Autodesk Inventor part; units mm, degrees
ref_plane "YZ Plane" through (0, 0, 0) normal (1, 0, 0) x (0, 1, 0)
ref_plane "XZ Plane" through (0, 0, 0) normal (0, 1, 0) x (-1, 0, 0)
ref_plane "XY Plane" through (0, 0, 0) normal (0, 0, 1) x (1, 0, 0)
sketch "Sketch1" plane through (0, 0, 0) normal (0, 0, 1) x (1, 0, 0)
  line L0 (0, 0) -> (22, 0)
  line L1 (22, 0) -> (22, 5)
  line L2 (22, 5) -> (0, 5)
  line L3 (0, 5) -> (0, 0)
  line L4 (22, 0) -> (13, 0)
  line L5 (13, 0) -> (13, 4)
  line L6 (13, 4) -> (22, 4)
  line L7 (22, 4) -> (22, 0)
  line L8 (13, 4) -> (13, 5)
  line L9 (22, 0) -> (0, 0)
  line L10 (0, 0) -> (0, 2.6)
  line L11 (0, 2.6) -> (22, 2.6)
  line L12 (22, 2.6) -> (22, 0)
  dimension "d0" = 22
  dimension "d1" = 5
  dimension "d2" = 9
  dimension "d3" = 4
  dimension "d4" = 2.6
revolve "Revolution1" add sketch "Sketch1" angle 360 about axis through (0, 0, 0) along (1, 0, 0) contours L3 L2 L8 L5 L11 | L5 L6 L1 L11
chamfer "Chamfer1" distance 1 angle 45 3 edges at (22, -2.6, 0) (0, -2.6, 0) (0, -5, 0)
properties part number "Vezetőhüvely"
Geometry check sheet. Reference: the model listing, model coordinates, mm. Give positions to 0.01 mm unless a question says otherwise; leave off trailing zeros. Order: outer loops, then holes, each group sorted by start corner. A loop starts at its lowest first (then second) coordinate and runs counter-clockwise, first axis right, second up. Notation, with made-up numbers: (63.5, -18.75) -> (81.5, -18.75) arc R20 cw to (81.5, 13.25) -> close; hole circle Ø5 at (56.25, 86). An arc over 180 degrees is marked (long way). Write each question's results on one line, items separated by ' | '. Start each with the question number.
(1) Scan lines: line 1 (Z direction, x = 6.75, y = 0); line 2 (Z direction, x = 13.5, y = 0); line 3 (Y direction, x = 10, z = 0.5). Record each from-to range of solid material in increasing order.
(2) Sectioned sample at D-D (x = 17.5). Enter the section's corners in (y, z).
(3) Sectioned sample at C-C (x = 4.25). Enter the section's corners in (y, z), plus the area to 3 significant figures.
(4) Sectioned sample at A-A (y = 0). Enter the section's corners in (x, z), plus the area to 3 significant figures.
(5) Mould release check, pull along Z, two halves, no side actions. Record for faces 1 (the face through (11.14, -0.338, 2.578)), 2 (the face through (6.92, -1.08, 4.88)): pulls with the +Z half, pulls with the -Z half, needs draft (parallel to the pull), parting line crosses it, or undercut.
(6) Gauge pin test, flat ends, axial feed: P1, Ø4, axis at x = 18, z = 1, coming from the -Y side; P2, Ø6, axis at x = 16.5, y = 2.5, coming from the +Z side; P3, Ø1.5, axis at x = 12.5, z = -2, coming from the +Y side; P4, Ø4.5, axis at y = 0, z = 0, coming from the -X side. Record the tip position at first contact, or that the pin passes through.
Answer below:
1) line 1: -5 to -2.6, 2.6 to 5 | line 2: -4 to -2.6, 2.6 to 4 | line 3: -4.97 to -2.55, 2.55 to 4.97
2) outline: circle Ø8 at (0, 0); hole circle Ø5.2 at (0, 0)
3) outline: circle Ø10 at (0, 0); hole circle Ø5.2 at (0, 0) | area: 57.3 mm2
4) outline: (0, -4) -> (1, -5) -> (13, -5) -> (13, -4) -> (22, -4) -> (22, -3.6) -> (21, -2.6) -> (1, -2.6) -> (0, -3.6) -> close; (0, 3.6) -> (1, 2.6) -> (21, 2.6) -> (22, 3.6) -> (22, 4) -> (13, 4) -> (13, 5) -> (1, 5) -> (0, 4) -> close | area: 84.6 mm2
5) face 1: undercut | face 2: parting line crosses it
6) P1: y = -4 | P2: z = 4 | P3: y = 4.84 | P4: through
